```python
from build123d import *

# Parameters (mm, degrees)
F0_W     = 17
F0_H     = 20
F0_R     = 3.57
F1_DEPTH = 4
F2_W     = 17
F2_H     = 16
F2_R     = 3.57
F3_DEPTH = 4


with BuildPart() as f1:
    # F0 (on Front) → F1 (new body)
    with BuildSketch(Plane.XZ):
        Rectangle(F0_W, F0_H)
        with Locations((0, 2.212742)):
            Circle(F0_R, mode=Mode.SUBTRACT)
    extrude(amount=F1_DEPTH)

    # F2 (on face) → F3 (join)
    with BuildSketch(Plane(origin=(0, 0, -10), x_dir=(1, 0, 0), z_dir=(0, 0, -1))):
        with Locations((0, -8)):
            Rectangle(F2_W, F2_H)
        with Locations((0, -7.547601)):
            Circle(F2_R, mode=Mode.SUBTRACT)
    extrude(amount=-F3_DEPTH)


solid = f1.part
```
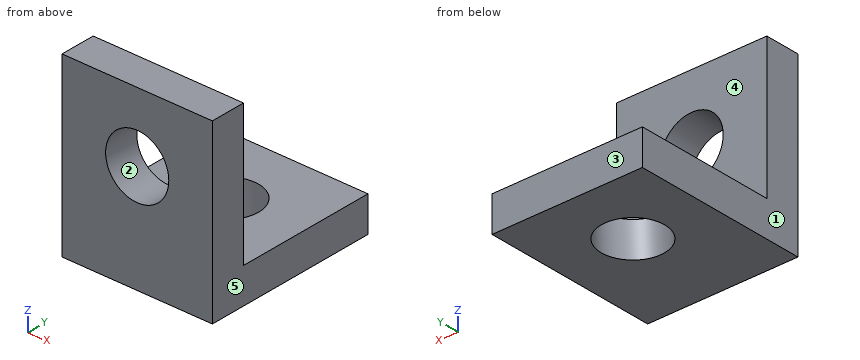
For this review, take the finished solid that the model builds, in its own axes (mm). Face numbers are marked on the shaded views. A direction names the side the tool comes from. Coordinates: 2 decimals unless noted, no trailing zeros. Write each loop counter-clockwise with the first axis right and the second up, starting at its lowest first coordinate (ties: lowest second). Pieces come first, ordered by that corner, then holes. Notation, with made-up numbers: (89, 83.25) - (112, 83.25) arc R11 ccw to (112, 103.25) - close; hole circle Ø6 at (77, 60). An arc over 180 degrees is marked (long way). Put each result on its own line as item: value.
1. Add section D-D, the plane x = -6.5. Give the boundary of the cut face in (y, z), then the cut area to 3 significant figures.
Values found:
outline: (-4, -10) - (16, -10) - (16, -6) - (0, -6) - (0, 10) - (-4, 10) - close
area: 144 mm²
2. Machinability: for the marked faces 4 and 5, which of the approach directions +Z, -Z, +X, -X, +Y, -Y give a long, thin tool a straight path to every point of the face, cutting with its end or side? Answer none if there is none.
Values found:
face 4: +Z, +X, -X, +Y
face 5: +Z, -Z, +X, +Y, -Y
3. Wall thickness on probe 1 along Z at (x, y) = (0, -2.7); probe 2 along Y at (x, z) = (0, -7.9); probe 3 along Y at (x, z) = (4, 9): over which ranges is each line inside the solid? List them lowest first.
Values found:
probe 1: -10 to -1.36, 5.78 to 10
probe 2: -4 to 3.98, 11.12 to 16
probe 3: -4 to 0
4. Add section C-C, the plane y = 5. Give the boundary of the cut face in (x, z).
Values found:
outline: (-8.5, -10) - (-2.5, -10) - (-2.5, -6) - (-8.5, -6) - close; (2.5, -10) - (8.5, -10) - (8.5, -6) - (2.5, -6) - close
5. For pin 1 (5 mm diameter, centred on x = 1, y = 8.5, fed in from +Z); pin 2 (9.5 mm diameter, centred on x = 0, z = 2.21, fed in from +Y), all flat-tipped, find the tip position at first contact; note any pin that passes through.
Values found:
pin 1: z = -6
pin 2: y = 0
6. Add section B-B, the plane z = -0.75. Give the boundary of the cut face in (x, y).
Values found:
outline: (-8.5, -4) - (-1.99, -4) - (-1.99, 0) - (-8.5, 0) - close; (1.99, -4) - (8.5, -4) - (8.5, 0) - (1.99, 0) - close
7. Add section A-A, the plane x = 2.5. Give the boundary of the cut face in (y, z).
Values found:
outline: (-4, -10) - (5, -10) - (5, -6) - (0, -6) - (0, -0.34) - (-4, -0.34) - close; (-4, 4.76) - (0, 4.76) - (0, 10) - (-4, 10) - close; (10.1, -10) - (16, -10) - (16, -6) - (10.1, -6) - close
8. Mouldability with a two-part tool opening along X and no side actions: class the marked faces 1, 2 and 3 as released by +X, released by -X, zero draft, split by the parting line, or undercut.
Values found:
face 1: released by -X
face 2: undercut
face 3: zero draft
